For this review, take the finished solid that the model builds, in its own axes (mm). Face numbers are marked on the shaded views. A direction names the side the tool comes from. Coordinates: 2 decimals unless noted, no trailing zeros. Write each loop counter-clockwise with the first axis right and the second up, starting at its lowest first coordinate (ties: lowest second). Pieces come first, ordered by that corner, then holes.
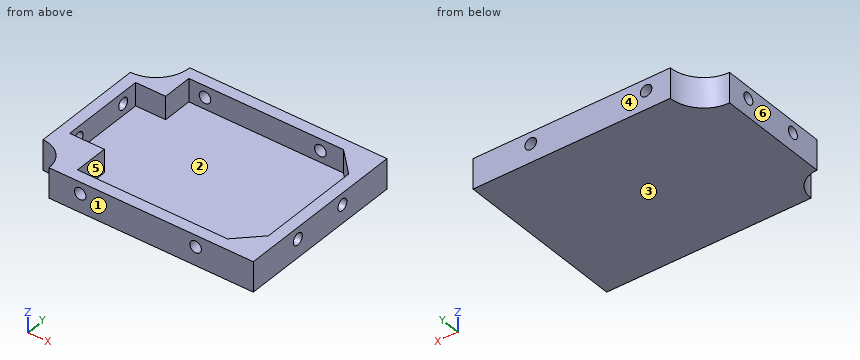
```python
from build123d import *

# Parameters (mm, degrees)
BOSS_EXTRU_1_DEPTH        = 13
COQUE1_T                  = -5
COQUE1_THICKNESS_2_FACE_W = 90
COQUE1_THICKNESS_2_FACE_H = 65
COQUE1_THICKNESS_2_DEPTH  = 2
ENL_V_MAT_EXTRU_1_REACH   = 110.96
ESQUISSE2_R               = 2.5
ENL_V_MAT_EXTRU_2_REACH   = 95.396
ESQUISSE3_R               = 2.5
ESQUISSE4_W               = 18
ESQUISSE4_H               = 18
ESQUISSE4_W_2             = 15
ESQUISSE4_H_2             = 15
BOSS_EXTRU_2_DEPTH        = 10
ESQUISSE6_R               = 11.5
ESQUISSE6_R_2             = 14.5
ENL_V_MAT_EXTRU_4_DEPTH   = 13


with BuildPart() as part:
    # Esquisse1 → Boss.-Extru.1 (new body)
    with BuildSketch(Plane.XY):
        Polygon((44.118436308, 33.728448276), (54.118436308, 33.728448276), (54.118436308, 23.728448276), (54.118436308, -41.271551724), (-45.881563692, -41.271551724), (-45.881563692, 33.728448276), align=None)
    extrude(amount=BOSS_EXTRU_1_DEPTH)

    # Coque1
    coque1_openings = [part.faces().sort_by_distance(p)[0] for p in [
        (4.118436308, -3.771551724, 13),
    ]]
    offset(amount=COQUE1_T, openings=coque1_openings, kind=Kind.INTERSECTION)

    # Coque1 thickness 2 face (on inner face of the shell) → Coque1 thickness 2 (cut)
    with BuildSketch(Plane(origin=(4.118436308, -3.771551724, 5), x_dir=(-1, 0, 0), z_dir=(0, 0, -1))):
        Rectangle(COQUE1_THICKNESS_2_FACE_W, COQUE1_THICKNESS_2_FACE_H)
    extrude(amount=COQUE1_THICKNESS_2_DEPTH, mode=Mode.SUBTRACT)

    # Enlèv. mat.-Extru.1: up to this face of the body (flat: up to its plane)
    enl_v_mat_extru_1_end = Plane(part.part.faces().sort_by_distance((54.118436308, -3.771551724, 6.5))[0])
    # Esquisse2 → Enlèv. mat.-Extru.1 (cut, up to the picked face)
    with BuildSketch(Plane.ZY.offset(45.881563692), mode=Mode.PRIVATE) as enl_v_mat_extru_1_sk1:
        with Locations(Location((8, -16.271551724, 0), (0, 0, 270))):
            Circle(ESQUISSE2_R)
    enl_v_mat_extru_1_tool1 = split(extrude(enl_v_mat_extru_1_sk1.sketch, amount=-ENL_V_MAT_EXTRU_1_REACH, mode=Mode.PRIVATE), bisect_by=enl_v_mat_extru_1_end, keep=Keep.BOTH, mode=Mode.PRIVATE)
    # Esquisse2 → Enlèv. mat.-Extru.1 (cut, up to the picked face)
    with BuildSketch(Plane.ZY.offset(45.881563692), mode=Mode.PRIVATE) as enl_v_mat_extru_1_sk2:
        with Locations(Location((8, 8.728448276, 0), (0, 0, 270))):
            Circle(ESQUISSE2_R)
    enl_v_mat_extru_1_tool2 = split(extrude(enl_v_mat_extru_1_sk2.sketch, amount=-ENL_V_MAT_EXTRU_1_REACH, mode=Mode.PRIVATE), bisect_by=enl_v_mat_extru_1_end, keep=Keep.BOTH, mode=Mode.PRIVATE)
    add(enl_v_mat_extru_1_tool1.solids().sort_by(Axis((-45.881564, -16.271552, 8), (1, 0, 0)))[0], mode=Mode.SUBTRACT)
    add(enl_v_mat_extru_1_tool2.solids().sort_by(Axis((-45.881564, 8.728448, 8), (1, 0, 0)))[0], mode=Mode.SUBTRACT)

    # Enlèv. mat.-Extru.2: up to this face of the body (flat: up to its plane)
    enl_v_mat_extru_2_end = Plane(part.part.faces().sort_by_distance((4.118436308, 33.728448276, 6.5))[0])
    # Esquisse3 → Enlèv. mat.-Extru.2 (cut, up to the picked face)
    with BuildSketch(Plane.XZ.offset(41.271551724), mode=Mode.PRIVATE) as enl_v_mat_extru_2_sk1:
        with Locations(Location((-20.881563692, 8, 0), (0, 0, 270))):
            Circle(ESQUISSE3_R)
    enl_v_mat_extru_2_tool1 = split(extrude(enl_v_mat_extru_2_sk1.sketch, amount=-ENL_V_MAT_EXTRU_2_REACH, mode=Mode.PRIVATE), bisect_by=enl_v_mat_extru_2_end, keep=Keep.BOTH, mode=Mode.PRIVATE)
    # Esquisse3 → Enlèv. mat.-Extru.2 (cut, up to the picked face)
    with BuildSketch(Plane.XZ.offset(41.271551724), mode=Mode.PRIVATE) as enl_v_mat_extru_2_sk2:
        with Locations(Location((29.118436308, 8, 0), (0, 0, 270))):
            Circle(ESQUISSE3_R)
    enl_v_mat_extru_2_tool2 = split(extrude(enl_v_mat_extru_2_sk2.sketch, amount=-ENL_V_MAT_EXTRU_2_REACH, mode=Mode.PRIVATE), bisect_by=enl_v_mat_extru_2_end, keep=Keep.BOTH, mode=Mode.PRIVATE)
    add(enl_v_mat_extru_2_tool1.solids().sort_by(Axis((-20.881564, -41.271552, 8), (0, 1, 0)))[0], mode=Mode.SUBTRACT)
    add(enl_v_mat_extru_2_tool2.solids().sort_by(Axis((29.118436, -41.271552, 8), (0, 1, 0)))[0], mode=Mode.SUBTRACT)

    # Esquisse4 → Boss.-Extru.2 (add)
    with BuildSketch(Plane.XY.offset(3)):
        with Locations((-36.881563692, 24.728448276)):
            Rectangle(ESQUISSE4_W, ESQUISSE4_H)
        Polygon((49.118436308, 28.728448276), (49.118436308, 18.728448276), (39.118436308, 28.728448276), align=None)
        Polygon((49.118436308, -36.271551724), (49.118436308, -26.271551724), (39.118436308, -36.271551724), align=None)
        with Locations((-33.381563692, -28.771551724)):
            Rectangle(ESQUISSE4_W_2, ESQUISSE4_H_2)
    extrude(amount=BOSS_EXTRU_2_DEPTH)

    # Esquisse6 → Enlèv. mat.-Extru.4 (cut)
    with BuildSketch(Plane.XY.offset(13)):
        with Locations((-45.881563692, -41.271551724)):
            Circle(ESQUISSE6_R)
        with Locations((-45.881563692, 33.728448276)):
            Circle(ESQUISSE6_R_2)
    extrude(amount=-ENL_V_MAT_EXTRU_4_DEPTH, mode=Mode.SUBTRACT)


solid = part.part
```
Q1. Clearance check with flat-ended pins moving along their axes: pin 1 Ø6.5 at (y, z) = (8.73, 8) entering from -X; pin 2 Ø4.5 at (x, z) = (29.12, 8) entering from -Y; pin 3 Ø3 at (x, y) = (7, -8) entering from +Z. State where each tip first meets the part, or that it passes through.
Ans:
pin 1: stops at x = -45.88
pin 2: passes through
pin 3: stops at z = 3
Q2. Add section B-B (x = 8.5). State the section outline as (y, z) points, then the cut area to 3 significant figures.
Ans:
outline: (-41.27, 0) - (33.73, 0) - (33.73, 13) - (28.73, 13) - (28.73, 3) - (-36.27, 3) - (-36.27, 13) - (-41.27, 13) - close
area: 325 mm2
Q3. Add section C-C (z = 8). Give the number of separate pieces and of enclosed holes in the cut face, then the cut area to 4 significant figures.
Ans:
separate pieces: 8
enclosed holes: 0
area: 1,675 mm2
Q4. For probe 1 along X at (y, z) = (-24, 6.75); probe 2 along X at (y, z) = (31.5, 8); probe 3 along X at (y, z) = (12, 4.75), list the stretches that pass through material, from the lowest coordinate up.
Ans:
probe 1: x = -45.88 to -25.88, 49.12 to 54.12
probe 2: x = -31.55 to -23.38, -18.38 to 26.62, 31.62 to 54.12
probe 3: x = -45.88 to -40.88, 49.12 to 54.12
Q5. Draft analysis for pull direction Y (two halves, no side actions). For the marked faces 1, 2, 3 and 4, state which applies: +Y half, -Y half, draft (parallel to the pull), parting line (faces both ways), or undercut.
Ans:
face 1: -Y half
face 2: undercut
face 3: draft
face 4: +Y half
Q6. Add section A-A (y = -5). State the section outline as (x, z) points.
Ans:
outline: (-45.88, 0) - (54.12, 0) - (54.12, 13) - (49.12, 13) - (49.12, 3) - (-40.88, 3) - (-40.88, 13) - (-45.88, 13) - close
Q7. Tool access review of the marked faces 5 and 6: name each direction out of +Z, -Z, +X, -X, +Y, -Y from which nothing blocks a thin tool from reaching the whole face with its end or side.
Ans:
face 5: +Z
face 6: +Z, -Z, -X, +Y, -Y
